from build123d import *

# Parameters (mm, degrees)
SKETCH_1_W          = 15
SKETCH_1_H          = 15
SKETCH_1_W_2        = 13
SKETCH_1_H_2        = 13
EXTRUDE_1_DEPTH     = 340
SKETCH_2_R          = 1.45
CUT_EXTRUDE_1_DEPTH = 341.413351677
SKETCH_3_R          = 1.45
CUT_EXTRUDE_2_DEPTH = 341.413351677


with BuildPart() as part:
    # 草图1 → 凸台-拉伸1 (new body)
    with BuildSketch(Plane(origin=(0, 0, 0), x_dir=(0, 0, -1), z_dir=(1, 0, 0))):
        Rectangle(SKETCH_1_W, SKETCH_1_H)
        Rectangle(SKETCH_1_W_2, SKETCH_1_H_2, mode=Mode.SUBTRACT)
    extrude(amount=EXTRUDE_1_DEPTH)

    # 草图2 → 切除-拉伸1 (cut, through all)
    with BuildSketch(Plane.XZ.offset(7.5)):
        with Locations(Location((160, 0, 0), (0, 0, 270))):
            Circle(SKETCH_2_R)
        with Locations(Location((180, 0, 0), (0, 0, 90))):
            Circle(SKETCH_2_R)
    extrude(amount=-CUT_EXTRUDE_1_DEPTH, mode=Mode.SUBTRACT)

    # 草图3 → 切除-拉伸2 (cut, through all)
    with BuildSketch(Plane(origin=(0, 7.5, 0), x_dir=(1, 0, 0), z_dir=(0, 1, 0))):
        with Locations(Location((180, 0, 0), (0, 0, 270))):
            Circle(SKETCH_3_R)
        with Locations(Location((160, 0, 0), (0, 0, 90))):
            Circle(SKETCH_3_R)
        with Locations(Location((20, 0, 0), (0, 0, 270))):
            Circle(SKETCH_3_R)
        with Locations(Location((30, 0, 0), (0, 0, 270))):
            Circle(SKETCH_3_R)
        with Locations(Location((10, 0, 0), (0, 0, 270))):
            Circle(SKETCH_3_R)
        with Locations(Location((330, 0, 0), (0, 0, 270))):
            Circle(SKETCH_3_R)
        with Locations(Location((310, 0, 0), (0, 0, 270))):
            Circle(SKETCH_3_R)
        with Locations(Location((320, 0, 0), (0, 0, 270))):
            Circle(SKETCH_3_R)
    extrude(amount=-CUT_EXTRUDE_2_DEPTH, mode=Mode.SUBTRACT)


solid = part.part
The listing builds one solid part. Answer for the finished solid, in the listing's coordinates (mm). A direction names the side the tool comes from. Coordinates: 2 decimals unless noted, no trailing zeros. Loops run counter-clockwise (first coordinate to the right, second up) from the corner with the lowest first, then second, coordinate; pieces in that order, holes last.
1) Flat-ended cylindrical pins translate along their axes: pin 1 Ø1.7 at (x, z) = (20, 0) entering from +Y; pin 2 Ø3.5 at (x, z) = (180, 0) entering from +Y. Find the tip coordinate at first contact, or state that the pin passes through.
2) Find section A-A on y = 1. Write down the section's boundary in (x, z).
3) Find section B-B on x = 129. Write down the section's boundary in (y, z).
4) Find the intervals of material crossed by L1, parallel to Z at x = 180, y = 7.3; L2, parallel to Y at x = 315.5, z = -4, in increasing order.
5) A tool of negligible diameter and unlimited length cuts with its end or side. For faces 1 (the face through (168, 0, -7.5)), 2 (the face through (168, 0, 6.5)), from which of +Z, -Z, +X, -X, +Y, -Y can it reach the whole face along a straight path? Write none if from no direction.
6) Determine the mould class of faces 3 (the face through (168, 7.5, 0)), 4 (the face through (340, 0, 7)), 5 (the face through (168, -7.5, 0)), 6 (the face through (168, -6.5, 0)) for opening direction Y: pulls with the +Y half, pulls with the -Y half, needs draft (parallel to the pull), parting line crosses it, or undercut.
Values:
1. pin 1: passes through
1. pin 2: stops at y = 7.5
2. outline: (0, -7.5) - (340, -7.5) - (340, -6.5) - (0, -6.5) - close; (0, 6.5) - (340, 6.5) - (340, 7.5) - (0, 7.5) - close
3. outline: (-7.5, -7.5) - (7.5, -7.5) - (7.5, 7.5) - (-7.5, 7.5) - close; hole (-6.5, -6.5) - (6.5, -6.5) - (6.5, 6.5) - (-6.5, 6.5) - close
4. L1: z = -7.5 to -1.45, 1.45 to 7.5
4. L2: y = -7.5 to -6.5, 6.5 to 7.5
5. face 1: -Z, +X, -X, +Y, -Y
5. face 2: +X, -X
6. face 3: pulls with the +Y half
6. face 4: needs draft
6. face 5: pulls with the -Y half
6. face 6: undercut
